Here's how the part is built. I have some questions about the finished solid (model axes, mm). A direction names the side the tool comes from. Round coordinates to 2 decimals unless told otherwise and drop trailing zeros. Loops run counter-clockwise (first coordinate to the right, second up) from the corner with the lowest first, then second, coordinate; pieces in that order, holes last. Notation, with made-up numbers: (84.5, 14) - (115.5, 14) arc R9 cw to (115.5, 21) - close; hole circle Ø8 at (-12.5, 79). An arc over 180 degrees is marked (long way). Answer as a JSON object with one key per item and string values. Group by question number.
1) Which directions (+Z, -Z, +X, -X, +Y, -Y) give clear straight access to the entire face, cutting with the end or side of a thin tool? Please do faces 4 (the face through (-19, -38.1, 2)), 5 (the face through (-26.723, -11.844, 7.649)), 6 (the face through (40, -50.8, 8)), 7 (the face through (38, -38.1, 8)), 8 (the face through (-72, -84.074, 8)).
2) Will these pins go through, and if not, where does the flat tip stop? P1, Ø1, axis at x = 34, z = 7.5, coming from the -Y side; P2, Ø1.6, axis at x = 40.5, z = 7.5, coming from the +Y side; P3, Ø10, axis at x = -45.5, y = -30, coming from the -Z side.
3) I want a section at B-B, the plane y = -19.05. Please give me the cut outline in (x, z).
4) I want a section at C-C, the plane z = 7.75. Give the number of separate pieces and of enclosed holes in the cut face, then the cut area to 3 significant figures.
5) If we mould it in two halves opening along X, with no side actions, what happens to faces 1 (the face through (-37.376, -0.764, 1.796)), 2 (the face through (-0.724, -0.764, 1.796)), 3 (the face through (34, -84.074, 8))? For each: pulls with the +X half, pulls with the -X half, needs draft (parallel to the pull), parting line crosses it, or undercut.
6) I want a section at D-D, the plane y = -63.5. Please give me the cut outline in (x, z).
7) If I drill on line 1 along Y through (x, z) = (-19.05, 3.5); line 2 along Y through (x, z) = (-19.05, 5), over which ranges is the centre line in solid material (lowest first)? Write a range as [from, to].
8) I want a section at A-A, the plane y = -49. Please give me the cut outline in (x, z), then the cut area to 3 significant figures.
from build123d import *

# Parameters (mm, degrees)
SKETCH1_W           = 38.1
SKETCH1_H           = 38.1
BOSS_EXTRUDE1_DEPTH = 9.2583
SKETCH2_R           = 6.35
CUT_EXTRUDE1_DEPTH  = 10.8458
SKETCH3_R           = 1.778
CUT_EXTRUDE2_DEPTH  = 10.8458
CIRPATTERN1_COUNT   = 4
SKETCH4_W           = 31.5468
SKETCH4_H           = 95.2246
BOSS_EXTRUDE2_DEPTH = 3.175
SKETCH5_W           = 38.1
SKETCH5_H           = 57.1246
BOSS_EXTRUDE3_DEPTH = 3.175
FILLET1_R           = 2.54
FILLET2_R           = 2.54
BOSS_EXTRUDE4_DEPTH = 3.175
CUT_EXTRUDE3_DEPTH  = 4.7625


with BuildPart() as part:
    # Sketch1 → Boss-Extrude1 (new body)
    with BuildSketch(Plane.XY):
        with Locations((-19.05, -19.05)):
            Rectangle(SKETCH1_W, SKETCH1_H)
    extrude(amount=BOSS_EXTRUDE1_DEPTH)

    # Sketch2 → Cut-Extrude1 (cut)
    with BuildSketch(Plane.XY.offset(9.2583)):
        with Locations((-19.05, -19.05)):
            Circle(SKETCH2_R)
    extrude(amount=-CUT_EXTRUDE1_DEPTH, mode=Mode.SUBTRACT)

    # Sketch3 → Cut-Extrude2 (cut)
    with BuildSketch(Plane.XY.offset(9.2583)):
        with Locations((-19.05, -9.271)):
            Circle(SKETCH3_R)
    cut_extrude2 = extrude(amount=-CUT_EXTRUDE2_DEPTH, mode=Mode.SUBTRACT)

    # CirPattern1: Cut-Extrude2 ×4 about axis
    cirpattern1_axis = Axis((-19.05, -19.05, 0), (0, 0, 1))
    for i in range(1, CIRPATTERN1_COUNT):
        add(cut_extrude2.rotate(cirpattern1_axis, i * 360 / CIRPATTERN1_COUNT), mode=Mode.SUBTRACT)

    # Sketch4 → Boss-Extrude2 (add)
    with BuildSketch(Plane.XY.offset(9.2583)):
        with Locations((-53.8734, -47.6123)):
            Rectangle(SKETCH4_W, SKETCH4_H)
        with Locations((15.7734, -47.6123)):
            Rectangle(SKETCH4_W, SKETCH4_H)
    extrude(amount=-BOSS_EXTRUDE2_DEPTH)

    # Sketch5 → Boss-Extrude3 (add)
    with BuildSketch(Plane(origin=(0, 0, 6.0833), x_dir=(-1, 0, 0), z_dir=(0, 0, -1))):
        with Locations((19.05, -66.6623)):
            Rectangle(SKETCH5_W, SKETCH5_H)
    extrude(amount=-BOSS_EXTRUDE3_DEPTH)

    # Fillet1
    fillet1_edges = [part.edges().sort_by_distance(p)[0] for p in [
        (-38.1, -38.1, 3.04165),
        (-38.1, 0, 3.04165),
        (0, 0, 3.04165),
        (0, -38.1, 3.04165),
    ]]
    fillet(fillet1_edges, radius=FILLET1_R)

    # Fillet2
    # the kernel refuses this fillet: 2.54 mm, written as the material it adds along each edge
    with BuildSketch(Plane(origin=(-38.1, -35.56, 6.0833), x_dir=(0, 0, -1), z_dir=(0, 1, 0)), Plane(origin=(-2.54, -38.1, 6.0833), x_dir=(0, 0, -1), z_dir=(-1, 0, 0))) as fillet2_piece_1:
        with BuildLine():
            CenterArc((FILLET2_R, FILLET2_R), FILLET2_R, 180, 90)
            Line((0, FILLET2_R), (0, 0))
            Line((0, 0), (FILLET2_R, 0))
        make_face()
    extrude(amount=33.02)
    with BuildSketch(Plane(origin=(0, -35.56, 6.0833), x_dir=(0, 0, -1), z_dir=(0, 1, 0))) as fillet2_piece_2:
        with BuildLine():
            CenterArc((FILLET2_R, -FILLET2_R), FILLET2_R, 90, 90)
            Line((0, -FILLET2_R), (0, 0))
            Line((0, 0), (FILLET2_R, 0))
        make_face()
    extrude(amount=33.02)
    with BuildSketch(Plane(origin=(-35.56, -2.54, 6.0833), x_dir=(0.5976672776328278, -0.8017442392976482, 0), z_dir=(-0.8017442392976482, -0.5976672776328278, 0))) as fillet2_piece_3_section:
        with BuildLine():
            CenterArc((2.54 + FILLET2_R, -FILLET2_R), FILLET2_R, 90, 90)
            Line((2.54 + FILLET2_R, 0), (2.54, 0))
            Line((2.54, 0), (2.54, -FILLET2_R))
        make_face()
    fillet2_piece_3 = revolve(axis=Axis((-35.56, -2.54, 6.0833), (0, 0, 1)), revolution_arc=233.296989237, mode=Mode.PRIVATE)
    fillet2_piece_3 = split(fillet2_piece_3, bisect_by=Plane(origin=(-37.464844957, 0, 5.291764105), z_dir=(0, -1, 0)), keep=Keep.TOP, mode=Mode.PRIVATE)
    add(fillet2_piece_3)
    with BuildSketch(Plane(origin=(-35.56, -35.56, 6.0833), x_dir=(0, -1, 0), z_dir=(1, 0, 0))) as fillet2_piece_4:
        with BuildLine():
            CenterArc((2.54 + FILLET2_R, FILLET2_R), FILLET2_R, 180, 90)
            Line((2.54 + FILLET2_R, 0), (2.54, 0))
            Line((2.54, 0), (2.54, FILLET2_R))
        make_face()
    revolve(axis=Axis((-35.56, -35.56, 6.0833), (0, 0, -1)), revolution_arc=90)
    with BuildSketch(Plane(origin=(-2.54, -35.56, 6.0833), x_dir=(0, -1, 0), z_dir=(-1, 0, 0))) as fillet2_piece_5:
        with BuildLine():
            CenterArc((2.54 + FILLET2_R, -FILLET2_R), FILLET2_R, 90, 90)
            Line((2.54 + FILLET2_R, 0), (2.54, 0))
            Line((2.54, 0), (2.54, -FILLET2_R))
        make_face()
    revolve(axis=Axis((-2.54, -35.56, 6.0833), (0, 0, 1)), revolution_arc=90)
    with BuildSketch(Plane(origin=(-2.54, -2.54, 6.0833), x_dir=(-0.5976672776328275, -0.8017442392976483, 0), z_dir=(0.8017442392976483, -0.5976672776328275, 0))) as fillet2_piece_6_section:
        with BuildLine():
            CenterArc((2.54 + FILLET2_R, FILLET2_R), FILLET2_R, 180, 90)
            Line((2.54, FILLET2_R), (2.54, 0))
            Line((2.54, 0), (2.54 + FILLET2_R, 0))
        make_face()
    fillet2_piece_6 = revolve(axis=Axis((-2.54, -2.54, 6.0833), (0, 0, -1)), revolution_arc=233.296989237, mode=Mode.PRIVATE)
    fillet2_piece_6 = split(fillet2_piece_6, bisect_by=Plane(origin=(-0.63515521, 0, 5.291763812), z_dir=(0, -1, 0)), keep=Keep.TOP, mode=Mode.PRIVATE)
    add(fillet2_piece_6)

    # Sketch6 → Boss-Extrude4 (add)
    with BuildSketch(Plane(origin=(0, 0, 6.0833), x_dir=(-1, 0, 0), z_dir=(0, 0, -1))):
        Polygon((-36.3728, -50.8), (-44.2468, -50.8), (-44.2468, -38.1), (-31.5468, -38.1), (-31.5468, -44.45), (-36.3728, -44.45), align=None)
        Polygon((-36.3728, -90.424), (-44.2468, -90.424), (-44.2468, -77.724), (-31.5468, -77.724), (-31.5468, -84.074), (-36.3728, -84.074), align=None)
    boss_extrude4 = extrude(amount=-BOSS_EXTRUDE4_DEPTH)

    # Mirror2: Boss-Extrude4 across plane
    add(boss_extrude4.mirror(Plane(origin=(-19.05, 0, 0), x_dir=(0, 0, 1), z_dir=(1, 0, 0))))

    # Sketch8 → Cut-Extrude3 (cut)
    with BuildSketch(Plane(origin=(0, 0, 6.0833), x_dir=(-1, 0, 0), z_dir=(0, 0, -1))):
        Polygon((-25.1968, -38.1), (19.2532, -38.1), (9.7282, -6.35), (-15.6718, -6.35), align=None)
    cut_extrude3 = extrude(amount=-CUT_EXTRUDE3_DEPTH, mode=Mode.SUBTRACT)

    # Mirror3: Cut-Extrude3 across plane
    add(cut_extrude3.mirror(Plane(origin=(-19.05, 0, 0), x_dir=(0, 0, 1), z_dir=(1, 0, 0))), mode=Mode.SUBTRACT)


solid = part.part
Outcome:
{
 "1": {"face 4": "-Z, +X, -X, -Y", "face 5": "+Z", "face 6": "+Z, -Z, +X", "face 7": "+Z, -Z, +X, +Y", "face 8": "+Z, -Z, -Y"},
 "2": {"P1": "y = -84.07", "P2": "y = -38.1", "P3": "z = 6.08"},
 "3": {"outline": "(-69.65, 6.08) - (-57.58, 6.08) - (-57.58, 9.26) - (-69.65, 9.26) - close; (-40.64, 6.08) arc R2.54 cw to (-38.1, 3.54) - (-38.1, 0) - (-30.61, 0) - (-30.61, 6.08) - close; (-27.05, 0) - (-25.4, 0) - (-25.4, 6.08) - (-27.05, 6.08) - close; (-12.7, 0) - (-11.05, 0) - (-11.05, 6.08) - (-12.7, 6.08) - close; (-7.49, 0) - (0, 0) - (0, 3.54) arc R2.54 cw to (2.54, 6.08) - (-7.49, 6.08) - close; (19.48, 6.08) - (31.55, 6.08) - (31.55, 9.26) - (19.48, 9.26) - close"},
 "4": {"separate pieces": "2", "enclosed holes": "3", "area": "7,800 mm^2"},
 "5": {"face 1": "pulls with the -X half", "face 2": "pulls with the +X half", "face 3": "undercut"},
 "6": {"outline": "(-69.65, 6.08) - (31.55, 6.08) - (31.55, 9.26) - (-69.65, 9.26) - close"},
 "7": {"line 1": "[-38.1, -30.61], [-27.05, -25.4], [-12.7, -11.05], [-7.49, 0]", "line 2": "[-38.56, -30.61], [-27.05, -25.4], [-12.7, -11.05], [-7.49, 0]"},
 "8": {"outline": "(-82.35, 6.08) - (-74.47, 6.08) - (-74.47, 9.26) - (-82.35, 9.26) - close; (-69.65, 6.08) - (31.55, 6.08) - (31.55, 9.26) - (-69.65, 9.26) - close; (36.37, 6.08) - (44.25, 6.08) - (44.25, 9.26) - (36.37, 9.26) - close", "area": "371 mm^2"}
}
